```python
from build123d import *

# Parameters (mm, degrees)
F1_DEPTH = 1
F2_R     = 3
F2_R_2   = 3.25
F3_DEPTH = 2.001
F4_DEPTH = 1


with BuildPart() as f1:
    # F0 (on Front) → F1 (new body, symmetric)
    with BuildSketch(Plane.XZ):
        with BuildLine():
            ThreePointArc((30, 0), (16.77051, 24.874686), (-11.25, 27.810744))
            Line((-11.25, 27.810744), (-16.999625, 25.484906))
            Line((-16.999625, 25.484906), (-29.082446, 20.597165))
            Line((-29.082446, 20.597165), (-80, 0))
            Line((-80, 0), (-80, -40))
            Line((-80, -40), (30, -40))
            Line((30, -40), (30, 0))
        make_face()
    extrude(amount=F1_DEPTH, both=True)

    # F2 (on face) → F3 (cut, through all)
    with BuildSketch(Plane.XZ.offset(1)):
        Circle(F2_R)
        with Locations((-31, 0)):
            Circle(F2_R_2)
    extrude(amount=-F3_DEPTH, mode=Mode.SUBTRACT)

    # F0 (on Front) → F4 (join, symmetric)
    with BuildSketch(Plane.XZ):
        with BuildLine():
            Line((-29.082446, 20.597165), (-16.999625, 25.484906))
            Line((-16.999625, 25.484906), (-31.112698, 39.59798))
            ThreePointArc((-31.112698, 39.59798), (-39.59798, 39.59798), (-39.59798, 31.112698))
            Line((-39.59798, 31.112698), (-29.082446, 20.597165))
        make_face()
    extrude(amount=F4_DEPTH, both=True)


solid = f1.part
```
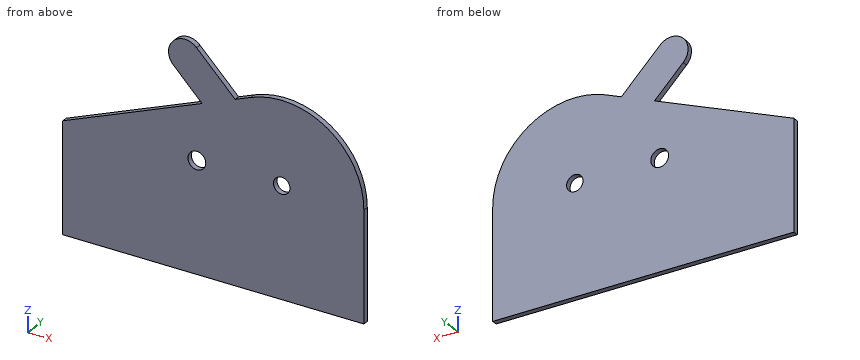
Model file for the job. Use its own axes, mm. Give positions to 0.01 mm unless a question says otherwise; leave off trailing zeros. Loops run counter-clockwise (first coordinate to the right, second up) from the corner with the lowest first, then second, coordinate; pieces in that order, holes last. Notation, with made-up numbers: M 68.5,2 L 98.5,2 A18 cw 98.5,32 Z; hole C -30.5,-15 d10. An arc over 180 degrees is marked long. Use one line per item in the form item = value.
Item 1: Slice it at B-B on y = -0.2. List the corners of the cut face in (x, z).
Filled in:
outline = M -80,-40 L 30,-40 L 30,0 A30 ccw -11.25,27.81 L -17,25.48 L -31.11,39.6 A6 ccw -39.6,31.11 L -29.08,20.6 L -80,0 Z; hole C -31,0 d6.5; hole C 0,0 d6
Item 2: Slice it at D-D on x = -49. List the corners of the cut face in (y, z).
Filled in:
outline = M -1,-40 L 1,-40 L 1,12.54 L -1,12.54 Z
Item 3: Flat gauge pin, fed straight in: pin 1 Ø5 at (x, z) = (0, 0) entering from -Y. Where does the tip first touch, or does it go through?
Filled in:
pin_1 = through
Item 4: Slice it at A-A on x = 0. List the corners of the cut face in (y, z), and give its area (3 significant figures).
Filled in:
outline = M -1,-40 L 1,-40 L 1,-3 L -1,-3 Z; M -1,3 L 1,3 L 1,30 L -1,30 Z
area = 128 mm^2
Item 5: Slice it at C-C on x = 20.5. List the corners of the cut face in (y, z).
Filled in:
outline = M -1,-40 L 1,-40 L 1,21.9 L -1,21.9 Z
Item 6: Drill centre lines: L1, parallel to Z at x = 0, y = -0.25; L2, parallel to Z at x = -32, y = -0.4; L3, parallel to Z at x = -31, y = 0.1. Where is each one in solid material? Low to high.
Filled in:
L1 = -40 to -3, 3 to 30
L2 = -40 to -3.09, 3.09 to 19.42, 23.51 to 40.33
L3 = -40 to -3.25, 3.25 to 19.82, 22.51 to 39.49
